Read the model definition and answer for the solid it produces. Units are mm, in the model's axes. A direction names the side the tool comes from. Coordinates: 2 decimals unless noted, no trailing zeros. Write each loop counter-clockwise with the first axis right and the second up, starting at its lowest first coordinate (ties: lowest second). Pieces come first, ordered by that corner, then holes.
from build123d import *

# Parameters (mm, degrees)
F2_DEPTH = 5
F3_R     = 4.99999
F5_D     = 5
F5_DEPTH = 17.5
F5_TIP   = 1.5021515476
F6_D     = 5
F6_DEPTH = 17.5
F6_TIP   = 1.5021515476


# Not quite as in the source:
# - a fillet or chamfer is up to 0.001 mm smaller than in the source, because OpenCascade refuses the exact size


with BuildPart() as f2:
    # F1 (on Top) → F2 (new body, symmetric)
    with BuildSketch(Plane.XY):
        with BuildLine():
            Line((27.5, 0), (17.5, 0))
            ThreePointArc((17.5, 0), (0, -17.5), (-17.5, 0))
            Line((-17.5, 0), (-27.5, 0))
            ThreePointArc((-27.5, 0), (0, -27.5), (27.5, 0))
        make_face()
        with BuildLine():
            ThreePointArc((-17.5, 0), (0, 17.5), (17.5, 0))
            Line((17.5, 0), (27.5, 0))
            Line((27.5, 0), (27.5, 27.5))
            Line((27.5, 27.5), (0, 27.5))
            Line((0, 27.5), (-27.5, 27.5))
            Line((-27.5, 27.5), (-27.5, 0))
            Line((-27.5, 0), (-17.5, 0))
        make_face()
    extrude(amount=F2_DEPTH, both=True)

    # F3 (radius 5 in the source; OpenCascade refuses exactly that, so slightly less here)
    f3_edges = [f2.edges().sort_by_distance(p)[0] for p in [
        (17.5, 0, -5),
        (0, -27.5, -5),
        (0, -27.5, 5),
        (17.5, 0, 5),
    ]]
    fillet(f3_edges, radius=F3_R)

    # F5
    with Locations(Plane(origin=(0, 27.5, 0), x_dir=(-1, 0, 0), z_dir=(0, 1, 0))):
        with Locations((-22.5, 0)):
            Hole(F5_D / 2, depth=F5_DEPTH)
            with Locations((0, 0, -(F5_DEPTH + F5_TIP / 2))):  # 118° drill point
                Cone(0, F5_D / 2, F5_TIP, mode=Mode.SUBTRACT)

    # F6
    with Locations(Plane(origin=(0, 27.5, 0), x_dir=(-1, 0, 0), z_dir=(0, 1, 0))):
        with Locations((22.5, 0)):
            Hole(F6_D / 2, depth=F6_DEPTH)
            with Locations((0, 0, -(F6_DEPTH + F6_TIP / 2))):  # 118° drill point
                Cone(0, F6_D / 2, F6_TIP, mode=Mode.SUBTRACT)


solid = f2.part
Item 1: The part is cut by section C-C (y = 20.5). State how many separate pieces and enclosed holes the cut face has, and give its area (3 significant figures).
Item 2: Find the intervals of material crossed by probe 1 along Y at (x, z) = (0, 0); probe 2 along X at (y, z) = (19.75, 0); probe 3 along Z at (x, y) = (-22.5, 14.5), in increasing order.
Item 3: The part is cut by section B-B (z = -4). Give the vertices of the cut face in (x, y).
Item 4: Given pin 1 (3 mm diameter, centred on y = -20, z = -3, fed in from -X); pin 2 (2 mm diameter, centred on y = 22, z = 3, fed in from +X), each flat-ended and moving along its own axis, determine where each tip first touches the part or whether it passes through.
Item 5: Determine the mould class of faces 1 (the cylindrical face through (20, 19, 0)), 2 (the flat face through (0, 23, -5)), 3 (the conical face through (-22.9, 8.76, -0.17)), 4 (the cylindrical face through (26.07, 13.94, 3.5)) for opening direction X: +X half, -X half, draft (parallel to the pull), parting line (faces both ways), or undercut.
Item 6: For faces 5 (the flat face through (0, 23, 5)), 6 (the cylindrical face through (-25, 19, 0)), determine the directions among +Z, -Z, +X, -X, +Y, -Y from which every point of the face is accessible in a straight line to the end or side of a thin tool.
Answer:
1. separate pieces: 1
1. enclosed holes: 2
1. area: 481 mm2
2. probe 1: y = -27.5 to -17.5, 17.5 to 27.5
2. probe 2: x = -27.5 to -25, -20 to 20, 25 to 27.5
2. probe 3: z = -5 to -2.5, 2.5 to 5
3. outline: (-25.5, 0) arc R25.5 ccw to (25.5, 0) - (25.5, 27.5) - (-25.5, 27.5) - close; hole circle Ø39 at (0, 0)
4. pin 1: stops at x = -19.43
4. pin 2: stops at x = 27.08
5. face 1: undercut
5. face 2: draft
5. face 3: undercut
5. face 4: +X half
6. face 5: +Z, +X, -X, +Y, -Y
6. face 6: +Y
